Geometry: final body of the model. Coordinates: model frame, mm. Face numbers are marked on the shaded views. A direction names the side the tool comes from. Round coordinates to 2 decimals unless told otherwise and drop trailing zeros. Write each loop counter-clockwise with the first axis right and the second up, starting at its lowest first coordinate (ties: lowest second). Pieces come first, ordered by that corner, then holes. Notation, with made-up numbers: M 30.5,-10 L 48.5,-10 A30 cw 48.5,21 Z; hole C 89,42 d11. An arc over 180 degrees is marked long. Answer as CSV lines item,"result". Start each with the question number.
Q1. Section query A-A on y = 10.8. Output: boundary loops of the cut face in (x, z), and give its area (3 significant figures).
Q2. Section query B-B on x = -10.5. Output: boundary loops of the cut face in (y, z).
Q3. Reachability of the marked faces 5, 6 and 7 from +Z, -Z, +X, -X, +Y, -Y: full face, straight path, thin tool, end or side. Return the list, or none.
Q4. Ray query, probe 1 along X at (y, z) = (3.75, 0); probe 2 along X at (y, z) = (15, -4.75); probe 3 along Y at (x, z) = (3.3, -5.25). Return the intervals inside material, ascending.
Q5. Section query D-D on z = 3.3. Output: boundary loops of the cut face in (x, y).
Q6. First-contact query: pin 1 (10 mm diameter, centred on x = -4, y = 26, fed in from +Z); pin 2 (1 mm diameter, centred on x = -9, z = 0, fed in from -Y); pin 3 (1.3 mm diameter, centred on y = 34.2, z = -3.3, fed in from -X). Flat tips, straight axial feed; report the tip coordinate or a pass-through.
Q7. Section query C-C on y = 17.5. Output: boundary loops of the cut face in (x, z), and give its area (3 significant figures).
Q8. Mould query, pull axis X, two halves, no side actions, for the marked faces 1, 2, 3 and 4. Classes: pulls with the +X half, pulls with the -X half, needs draft (parallel to the pull), parting line crosses it, or undercut.
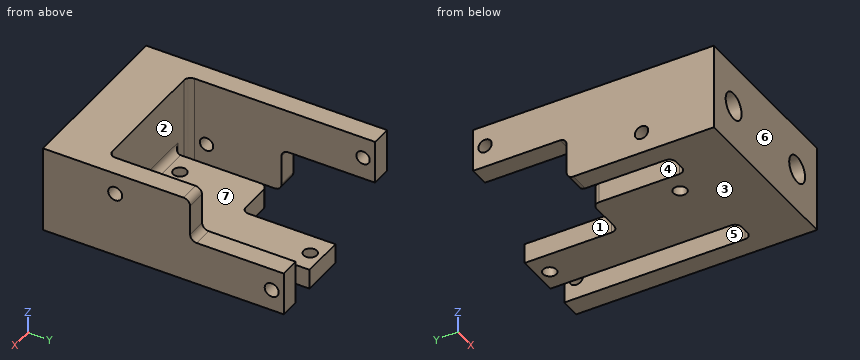
Autodesk Inventor part; units mm, degrees
ref_plane "TOP" through (0, 36, 0) normal (0, 1, 0) x (-1, 0, 0)
ref_plane "Work Plane2" through (13, 22, 6.5) normal (0, 1, 0) x (1, 0, 0)
ref_plane "YZ Plane" through (0, 0, 0) normal (1, 0, 0) x (0, 1, 0)
ref_plane "TOP" through (0, 36, 0) normal (0, 1, 0) x (-1, 0, 0)
sketch "Sketch1" plane through (0, 0, 0) normal (0, 1, 0) x (-1, 0, 0)
  line L0 (13, -6.5) -> (-13, -6.5)
  line L1 (-13, -6.5) -> (-13, 6.5)
  line L2 (-13, 6.5) -> (13, 6.5)
  line L3 (13, 6.5) -> (13, -6.5)
  line L4 (0, -9.1) -> (0, 9.1)
  line L5 (18.2, 0) -> (-18.2, 0)
  point P0 (0, 0)
  dimension "d0" = 26
  dimension "d1" = 13
extrude "Extrusion1" add sketch "Sketch1" along normal blind 8
sketch "Sketch2" plane through (0, 8, 0) normal (0, 1, 0) x (1, 0, 0)
  line L0 (-13, 6.5) -> (-13, -6.5)
  line L1 (-13, 6.5) -> (-10, 6.5)
  line L2 (-10, 6.5) -> (-10, -6.5)
  line L3 (-10, -6.5) -> (-13, -6.5)
  line L4 (-13, -6.5) -> (-13, 6.5)
  line L5 (13, 6.5) -> (-13, 6.5)
  line L6 (13, 6.5) -> (10, 6.5)
  line L7 (10, 6.5) -> (10, -6.5)
  line L8 (10, -6.5) -> (13, -6.5)
  line L9 (13, -6.5) -> (13, 6.5)
  line L10 (-6.5, 6.5) -> (6.5, 6.5)
  line L11 (6.5, 6.5) -> (6.5, 3.5)
  line L12 (6.5, 3.5) -> (-6.5, 3.5)
  line L13 (-6.5, 3.5) -> (-6.5, 6.5)
  line L14 (0, 9.1) -> (0, -9.1)
  line L15 (-13, -6.5) -> (13, -6.5)
  point P0 (0, 0)
  dimension "d4" = 3
  dimension "d5" = 3
  dimension "d6" = 3
  dimension "d7" = 13
extrude "Extrusion2" add sketch "Sketch2" along normal up to surface (28 mm away) contours L1 L2 L3 L0 | L5 L14 L12 L13 | L5 L11 L12 L14 | L7 L5 L9 L8
sketch "Sketch3" plane through (-13, 0, -6.5) normal (-1, 0, 0) x (0, 0, 1)
  line L0 (0, 36) -> (6.5, 36)
  line L1 (6.5, 36) -> (6.5, 22)
  line L2 (6.5, 22) -> (0, 22)
  line L3 (0, 22) -> (0, 36)
  line L4 (0, 0) -> (13, 0)
  line L5 (13, 0) -> (13, 36)
  line L6 (13, 36) -> (0, 36)
  line L7 (0, 0) -> (0, 36)
  point P0 (6.5, 0)
  dimension "d11" = 22
  dimension "d12" = 6.5
extrude "Extrusion3" cut sketch "Sketch3" against normal blind 3 contours L0 L1 L2 L3
sketch "Sketch4" plane through (13, 0, 6.5) normal (1, 0, 0) x (0, 0, -1)
  line L0 (6.5, 36) -> (0, 36)
  line L1 (0, 36) -> (6.5, 36)
  line L2 (6.5, 36) -> (6.5, 22)
  line L3 (6.5, 22) -> (0, 22)
  line L4 (0, 22) -> (0, 36)
  line L5 (-2.6, 0) -> (15.6, 0)
  line L6 (13, 0) -> (13, 36)
  point P0 (6.5, 0)
  dimension "d15" = 22
  dimension "d16" = 6.5
extrude "Extrusion4" cut sketch "Sketch4" against normal blind 3
sketch "Sketch5" plane through (-6.5, 8, -3.5) normal (0, 0, 1) x (1, 0, 0)
  line L0 (0, 0) -> (0, 28)
  line L1 (0, 28) -> (6.5, 28)
  line L2 (6.5, 28) -> (6.5, 14)
  line L3 (6.5, 14) -> (0, 14)
  line L4 (0, 14) -> (0, 28)
  line L5 (13, 0) -> (13, 28)
  line L6 (-6.5, -8) -> (19.5, -8)
  point P0 (6.5, -8)
  point P1 (0, 14)
  dimension "d19" = 6.5
  dimension "d20" = 22
extrude "Extrusion5" cut sketch "Sketch5" against normal blind 3
sketch "Sketch6" plane through (13, 0, 6.5) normal (1, 0, 0) x (0, 0, -1)
  circle A0 centre (9.8, 34.2) radius 1.05
  circle A1 centre (3.2, 10.8) radius 1.05
  line L0 (13, 0) -> (13, 36)
  line L1 (13, 36) -> (6.5, 36)
  line L2 (0, 0) -> (0, 22)
  line L3 (6.5, 36) -> (6.5, 22)
  point P0 (6.5, 0)
  point P1 (0, 8)
  dimension "d23" = 2.1
  dimension "d25" = 1.8
  dimension "d27" = 2.8
  dimension "d30" = 3.3
  dimension "d31" = 3.3
extrude "Extrusion6" cut sketch "Sketch6" against normal blind 3
ref_plane "Work Plane2" through (13, 22, 6.5) normal (0, 1, 0) x (1, 0, 0)
sketch "Sketch7" plane through (-13, 0, -6.5) normal (-1, 0, 0) x (0, 0, 1)
  circle A0 centre (9.8, 34.2) radius 1
  circle A1 centre (3.2, 10.8) radius 1
  line L0 (6.5, 43.2) -> (6.5, -7.2)
  line L1 (13, 36) -> (6.5, 36)
  line L2 (13, 8) -> (0, 8)
  line L3 (0, 8) -> (3, 8)
  line L4 (3, 8) -> (0, 8)
  line L5 (0, 8) -> (13, 8)
  point P0 (6.5, 0)
  dimension "d33" = 2
  dimension "d34" = 3.3
  dimension "d35" = 1.8
  dimension "d36" = 3.3
  dimension "d37" = 2.8
extrude "Extrusion7" cut sketch "Sketch7" against normal blind 3
sketch "Sketch8" plane through (-6.5, 8, -3.5) normal (0, 0, 1) x (1, 0, 0)
  circle A0 centre (9.8, 26.2) radius 1
  circle A1 centre (3.2, 2.8) radius 1
  line L0 (-11.7, 28) -> (24.7, 28)
  line L1 (6.5, 35.2) -> (6.5, -15.2)
  line L2 (-3.5, 0) -> (16.5, 0)
  point P0 (6.5, -8)
  dimension "d40" = 2
  dimension "d41" = 1.8
  dimension "d42" = 3.3
  dimension "d43" = 3.3
  dimension "d44" = 2.8
extrude "Extrusion8" cut sketch "Sketch8" against normal blind 3
sketch "Sketch9" plane through (0, 0, 0) normal (0, -1, 0) x (1, 0, 0)
  circle A0 centre (-8, 0) radius 2
  circle A1 centre (8, 0) radius 2
  line L0 (0, -9.1) -> (0, 9.1)
  line L1 (-18.2, 0) -> (18.2, 0)
  point P0 (0, 0)
  dimension "d47" = 4
  dimension "d48" = 16
extrude "Extrusion9" cut sketch "Sketch9" against normal blind 6
fillet "Fillet1" radius 1 11 edges at (10, 8, 0) (-10, 8, 0) (11.5, 22, 6.5) (11.5, 22, 0) (-11.5, 22, -6.5) (-11.5, 22, 0) (-6.5, 22, -5) (0, 22, -5) (6.5, 8, -5) (0, 8, -3.5) (-6.5, 8, -5)
properties part number "sg_sensor_mount"
Entries:
1,outline,"M -13,-6.5 L -10,-6.5 L -10,-4.3 L -13,-4.3 Z; M -13,-2.3 L -10,-2.3 L -10,6.5 L -13,6.5 Z; M -6.5,-6.5 L -4.3,-6.5 L -4.3,-3.5 L -6.5,-3.5 Z; M -2.3,-6.5 L 6.5,-6.5 L 6.5,-3.5 L -2.3,-3.5 Z; M 10,-6.5 L 13,-6.5 L 13,2.25 L 10,2.25 Z; M 10,4.35 L 13,4.35 L 13,6.5 L 10,6.5 Z"
1,area,"98.7 mm^2"
2,outline,"M 0,-6.5 L 21,-6.5 A1 ccw 22,-5.5 L 22,-1 A1 cw 23,0 L 36,0 L 36,6.5 L 0,6.5 Z; hole C 10.8,-3.3 d2; hole C 34.2,3.3 d2"
3,face 5,"+Z, -Z, +Y"
3,face 6,"+Z, -Z, +X, -X, -Y"
3,face 7,"+Z, +Y"
4,probe 1,"x = -13 to -10, -6 to 6, 10 to 13"
4,probe 2,"x = -13 to -10, -6.5 to 6.5, 10 to 13"
4,probe 3,"y = 0 to 33.2, 35.2 to 36"
5,outline,"M -13,0 L 13,0 L 13,9.75 L 10,9.75 L 10,9 A1 cw 9,8 L -9,8 A1 cw -10,9 L -10,33.2 L -13,33.2 Z; M -13,35.2 L -10,35.2 L -10,36 L -13,36 Z; M 10,11.85 L 13,11.85 L 13,22 L 10,22 Z"
6,pin 1,"stops at z = -3.5"
6,pin 2,"stops at y = 6"
6,pin 3,"stops at x = 0"
7,outline,"M -13,-6.5 L -10,-6.5 L -10,6.5 L -13,6.5 Z; M -6.5,-6.5 L 6.5,-6.5 L 6.5,-3.5 L -6.5,-3.5 Z; M 10,-6.5 L 13,-6.5 L 13,6.5 L 10,6.5 Z"
7,area,"117 mm^2"
8,face 1,"pulls with the -X half"
8,face 2,"undercut"
8,face 3,"needs draft"
8,face 4,"undercut"
